Print and shaded views of the part. All mm, measured from the part's lowest x, y and z. A direction names the side the tool comes from. Round coordinates to 2 decimals unless told otherwise and drop trailing zeros. Order: outer loops, then holes, each group sorted by start corner. A loop starts at its lowest first (then second) coordinate and runs counter-clockwise, first axis right, second up. Notation, with made-up numbers: (43, 72.5) - (80, 72.5) arc R11 cw to (80, 79.5) - close; hole circle Ø10 at (25, -21). An arc over 180 degrees is marked (long way). Write item = value, one per line.
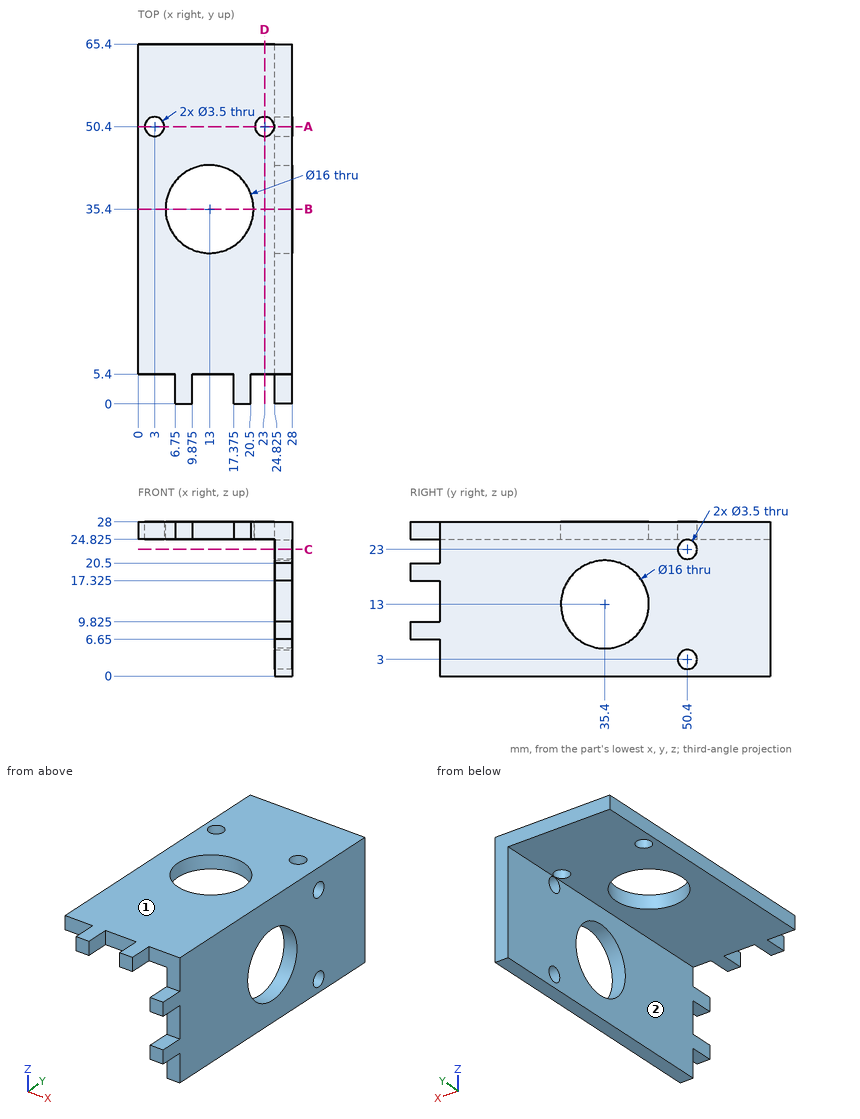
(1) Band-saw the part on A-A on y = 50.4. List the corners of the cut face in (x, z) (3 decimals), plus the area to 3 significant figures.
Solved:
outline = (0, 24.825) - (1.25, 24.825) - (1.25, 28) - (0, 28) - close; (4.75, 24.825) - (21.25, 24.825) - (21.25, 28) - (4.75, 28) - close; (24.75, 24.825) - (24.825, 24.825) - (24.825, 24.75) - (28, 24.75) - (28, 28) - (24.75, 28) - close; (24.825, 0) - (28, 0) - (28, 1.25) - (24.825, 1.25) - close; (24.825, 4.75) - (28, 4.75) - (28, 21.25) - (24.825, 21.25) - close
area = 123 mm²
(2) Drop flat-ended pins along their axis: pin 1 (2.5 mm diameter, centred on x = 4, z = 27, fed in from -Y); pin 2 (1.6 mm diameter, centred on y = 2, z = 26, fed in from -X); pin 3 (12.5 mm diameter, centred on x = 11.5, y = 25.5, fed in from -Z) (3 decimals). Give the stop position or say it passes through.
Solved:
pin_1 = 5.4
pin_2 = 6.75
pin_3 = 24.825
(3) Band-saw the part on C-C on z = 23. List the corners of the cut face in (x, y) (3 decimals), plus the area to 3 significant figures.
Solved:
outline = (24.825, 5.4) - (28, 5.4) - (28, 48.65) - (24.825, 48.65) - close; (24.825, 52.15) - (28, 52.15) - (28, 65.4) - (24.825, 65.4) - close
area = 179 mm²
(4) Tool access for the marked faces 1 and 2: list every direction of +Z, -Z, +X, -X, +Y, -Y with a clear straight run to the whole face (end or side of a thin tool).
Solved:
face_1 = +Z, +X, -X, +Y, -Y
face_2 = -Z, -X, +Y, -Y
(5) Probe line 1 along Y through (x, z) = (26.75, 3); line 2 along X through (y, z) = (62, 9) (3 decimals). List the from-to ranges inside material, lowest first.
Solved:
line_1 = 5.4 to 48.65, 52.15 to 65.4
line_2 = 24.825 to 28
(6) Band-saw the part on D-D on x = 23. List the corners of the cut face in (y, z) (3 decimals).
Solved:
outline = (5.4, 24.825) - (48.65, 24.825) - (48.65, 28) - (5.4, 28) - close; (52.15, 24.825) - (65.4, 24.825) - (65.4, 28) - (52.15, 28) - close
(7) Band-saw the part on B-B on y = 35.4. List the corners of the cut face in (x, z) (3 decimals), plus the area to 3 significant figures.
Solved:
outline = (0, 24.825) - (5, 24.825) - (5, 28) - (0, 28) - close; (21, 24.825) - (24.825, 24.825) - (24.825, 21) - (28, 21) - (28, 28) - (21, 28) - close; (24.825, 0) - (28, 0) - (28, 5) - (24.825, 5) - close
area = 66.1 mm²
